from build123d import *

# Parameters (mm, degrees)
SKETCH1_W            = 60
SKETCH1_H            = 60
SKETCH1_R            = 8
BOSS_EXTRUDE1_DEPTH  = 3
SKETCH2_R            = 1.5
CUT_EXTRUDE1_DEPTH   = 4
LPATTERN1_COUNT      = 2
LPATTERN1_PITCH      = 31
LPATTERN1_COUNT_DIR2 = 2
LPATTERN1_PITCH_DIR2 = 31
SKETCH3_R            = 2.5
CUT_EXTRUDE2_DEPTH   = 4
LPATTERN2_COUNT      = 3
LPATTERN2_PITCH      = 20
FILLET1_R            = 5


with BuildPart() as part:
    # Sketch1 → Boss-Extrude1 (new body)
    with BuildSketch(Plane(origin=(0, 0, 0), x_dir=(1, 0, 0), z_dir=(0, 1, 0))):
        with Locations((0, -10)):
            Rectangle(SKETCH1_W, SKETCH1_H)
        Circle(SKETCH1_R, mode=Mode.SUBTRACT)
    extrude(amount=BOSS_EXTRUDE1_DEPTH)

    # Sketch2 → Cut-Extrude1 (cut, through all)
    with BuildSketch(Plane(origin=(0, 3, 0), x_dir=(1, 0, 0), z_dir=(0, 1, 0))):
        with Locations((-15.5, 15.5)):
            Circle(SKETCH2_R)
    cut_extrude1 = extrude(amount=-CUT_EXTRUDE1_DEPTH, mode=Mode.SUBTRACT)

    # LPattern1: Cut-Extrude1 2 × 2
    with Locations(*[(i * LPATTERN1_PITCH, 0, j * LPATTERN1_PITCH_DIR2) for i in range(LPATTERN1_COUNT) for j in range(LPATTERN1_COUNT_DIR2) if (i, j) != (0, 0)]):
        add(cut_extrude1, mode=Mode.SUBTRACT)

    # Sketch3 → Cut-Extrude2 (cut, through all)
    with BuildSketch(Plane(origin=(0, 3, 0), x_dir=(1, 0, 0), z_dir=(0, 1, 0))):
        with Locations((-20, -30)):
            Circle(SKETCH3_R)
    cut_extrude2 = extrude(amount=-CUT_EXTRUDE2_DEPTH, mode=Mode.SUBTRACT)

    # LPattern2: Cut-Extrude2 ×3
    with Locations(*[(i * LPATTERN2_PITCH, 0, 0) for i in range(1, LPATTERN2_COUNT)]):
        add(cut_extrude2, mode=Mode.SUBTRACT)

    # Fillet1
    fillet1_edges = [part.edges().sort_by_distance(p)[0] for p in [
        (-30, 1.5, 40),
        (-30, 1.5, -20),
        (30, 1.5, -20),
        (30, 1.5, 40),
    ]]
    fillet(fillet1_edges, radius=FILLET1_R)


solid = part.part
Can you work these out from the model? Positions are in its coordinate system, mm. Round coordinates to 2 decimals unless told otherwise and drop trailing zeros. Write each loop counter-clockwise with the first axis right and the second up, starting at its lowest first coordinate (ties: lowest second). Pieces come first, ordered by that corner, then holes. Notation, with made-up numbers: (48, 65) -> (99, 65) arc R24 cw to (99, 100) -> close; hole circle Ø7 at (-35.75, 69). An arc over 180 degrees is marked (long way). Use one line per item in the form item = value. Start each with the question number.
Q1. If I drill on probe 1 along Z at (x, y) = (0, 0.75); probe 2 along Z at (x, y) = (15.5, 1.7); probe 3 along X at (y, z) = (2.1, 0), over which ranges is the centre line in solid material (lowest first)? Write a range as [from, to].
Q2. We'd pull the mould along X, two halves only. Please class faces 1 (the face through (28, 2, 39)), 2 (the face through (-29, 2, 38)), 3 (the face through (-21.84, 1.52, 28.31)): +X half, -X half, draft (parallel to the pull), parting line (faces both ways), or undercut.
Q3. Imagine slicing it at C-C (x = 18.5). Please give me the cut outline in (y, z).
Q4. Imagine slicing it at D-D (z = 15.5). Please give me the cut outline in (x, y), then the cut area to 3 significant figures.
Q5. Imagine slicing it at A-A (z = 30). Please give me the cut outline in (x, y), then the cut area to 3 significant figures.
Q6. Imagine slicing it at B-B (x = -15.5). Please give me the cut outline in (y, z).
Worked out:
q1.probe_1 = [-20, -8], [8, 27.5], [32.5, 40]
q1.probe_2 = [-20, -17], [-14, 14], [17, 40]
q1.probe_3 = [-30, -8], [8, 30]
q2.face_1 = +X half
q2.face_2 = -X half
q2.face_3 = undercut
q3.outline = (0, -20) -> (3, -20) -> (3, 28) -> (0, 28) -> close; (0, 32) -> (3, 32) -> (3, 40) -> (0, 40) -> close
q4.outline = (-30, 0) -> (-17, 0) -> (-17, 3) -> (-30, 3) -> close; (-14, 0) -> (14, 0) -> (14, 3) -> (-14, 3) -> close; (17, 0) -> (30, 0) -> (30, 3) -> (17, 3) -> close
q4.area = 162 mm^2
q5.outline = (-30, 0) -> (-22.5, 0) -> (-22.5, 3) -> (-30, 3) -> close; (-17.5, 0) -> (-2.5, 0) -> (-2.5, 3) -> (-17.5, 3) -> close; (2.5, 0) -> (17.5, 0) -> (17.5, 3) -> (2.5, 3) -> close; (22.5, 0) -> (30, 0) -> (30, 3) -> (22.5, 3) -> close
q5.area = 135 mm^2
q6.outline = (0, -20) -> (3, -20) -> (3, -17) -> (0, -17) -> close; (0, -14) -> (3, -14) -> (3, 14) -> (0, 14) -> close; (0, 17) -> (3, 17) -> (3, 40) -> (0, 40) -> close
